Verification items for the finished model (mm, model axes). Round coordinates to 2 decimals unless told otherwise and drop trailing zeros. Order: outer loops, then holes, each group sorted by start corner. A loop starts at its lowest first (then second) coordinate and runs counter-clockwise, first axis right, second up. Notation, with made-up numbers: (14, 8.5) -> (63, 8.5) arc R18 ccw to (63, 22.5) -> close; hole circle Ø1 at (20, 17). An arc over 180 degrees is marked (long way). Return JSON: item names as keys, results as strings. Group by question number.
1) Depth check by flat-ended pin: pin 1 (6 mm diameter, centred on x = 1, y = 6.5, fed in from -Z). Enter the tip coordinate at first touch or a pass-through.
2) Scan lines: L1, parallel to Y at x = 29.5, z = 119; L2, parallel to X at y = 7, z = 149; L3, parallel to Y at x = -34.5, z = 177.5. Record each from-to range of solid material in increasing order.
3) Section check A-A on x = 24.5. Enter the section's corners in (y, z), plus the area to 3 significant figures.
4) Section check B-B on z = 142. Enter the section's corners in (x, y).
Autodesk Inventor part; units mm, degrees
ref_plane "YZ Plane" through (0, 0, 0) normal (1, 0, 0) x (0, 1, 0)
ref_plane "XZ Plane" through (0, 0, 0) normal (0, 1, 0) x (-1, 0, 0)
ref_plane "XY Plane" through (0, 0, 0) normal (0, 0, 1) x (1, 0, 0)
sketch "Sketch1" plane through (0, 0, 0) normal (0, 0, 1) x (1, 0, 0)
  line L0 (-60, 30) -> (60, 30)
  line L1 (60, 30) -> (60, 0)
  line L2 (60, 0) -> (30, 0)
  line L3 (30, 0) -> (36, 10)
  line L4 (36, 10) -> (-36, 10)
  line L5 (-36, 10) -> (-30, 0)
  line L6 (-30, 0) -> (-60, 0)
  line L7 (-60, 0) -> (-60, 30)
  line L8 (0, 0) -> (0, 10) construction
  line L9 (0, 10) -> (0, 30) construction
  dimension "d0" = 30
  dimension "d1" = 20
  dimension "d2" = 72
  dimension "d3" = 6
  dimension "d4" = 6
  dimension "d5" = 120
  dimension "d6" = 30
extrude "Extrusion1" add sketch "Sketch1" along normal blind 210
chamfer "Chamfer1" distance 2 angle 45 8 edges at (60, 15, 210) (60, 30, 105) (0, 30, 210) (-60, 15, 210) (-60, 30, 105) (-60, 15, 0) (0, 30, 0) (60, 15, 0)
properties part number "Cross Slide"
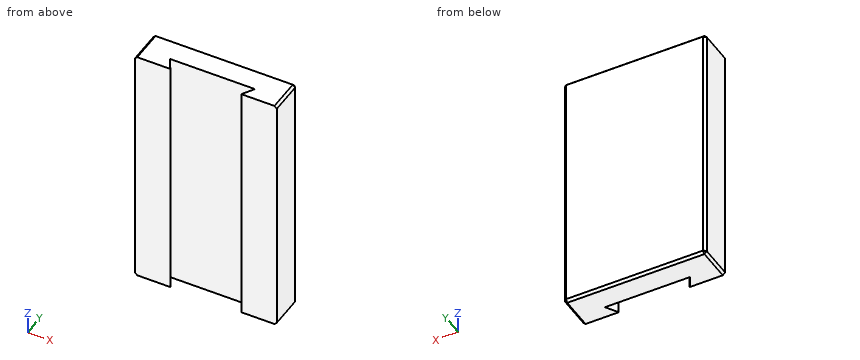
Check result:
{
 "1": {"pin 1": "through"},
 "2": {"L1": "10 to 30", "L2": "-60 to -34.2, 34.2 to 60", "L3": "0 to 7.5, 10 to 30"},
 "3": {"outline": "(10, 0) -> (28, 0) -> (30, 2) -> (30, 208) -> (28, 210) -> (10, 210) -> close", "area": "4,200 mm^2"},
 "4": {"outline": "(-60, 0) -> (-30, 0) -> (-36, 10) -> (36, 10) -> (30, 0) -> (60, 0) -> (60, 28) -> (58, 30) -> (-58, 30) -> (-60, 28) -> close"}
}
